from build123d import *

# Parameters (mm, degrees)
SKETCH1_W           = 150
SKETCH1_H           = 120
BOSS_EXTRUDE1_DEPTH = 100
FILLET1_R           = 10
SHELL1_START        = -65
SHELL1_OUTLINE_W    = 90
SHELL1_OUTLINE_H    = 100
SHELL1_DEPTH        = 130
FILLET2_R           = 10
CUT_EXTRUDE1_DEPTH  = 37.5
BOSS_EXTRUDE2_START = 90
BOSS_EXTRUDE2_DEPTH = 90
SKETCH3_W           = 114.3
SKETCH3_H           = 50.8
CUT_EXTRUDE2_DEPTH  = 5.5
FILLET3_R           = 10


# Read off the part's stored shape, not the designer's step: Shell1
with BuildPart() as part:
    # Sketch1 → Boss-Extrude1 (new body)
    with BuildSketch(Plane(origin=(0, 0, 0), x_dir=(1, 0, 0), z_dir=(0, 1, 0))):
        Rectangle(SKETCH1_W, SKETCH1_H)
    extrude(amount=BOSS_EXTRUDE1_DEPTH)

    # Fillet1
    fillet1_edges = [part.edges().sort_by_distance(p)[0] for p in [
        (0, 0, 60),
        (-75, 0, 0),
        (0, 0, -60),
        (75, 0, 0),
        (75, 50, 60),
        (-75, 50, 60),
        (-75, 50, -60),
        (75, 50, -60),
    ]]
    fillet(fillet1_edges, radius=FILLET1_R)

    # Shell1 outline → Shell1 (cut)
    with BuildSketch(Plane.YZ.offset(SHELL1_START)):
        with Locations((55, 0)):
            Rectangle(SHELL1_OUTLINE_W, SHELL1_OUTLINE_H)
    extrude(amount=SHELL1_DEPTH, mode=Mode.SUBTRACT)

    # Fillet2
    fillet2_edges = [part.edges().sort_by_distance(p)[0] for p in [
        (65, 55, -50),
        (-65, 55, -50),
        (-65, 55, 50),
        (65, 55, 50),
    ]]
    fillet(fillet2_edges, radius=FILLET2_R)

    # Sketch2 → Cut-Extrude1 (cut, symmetric)
    with BuildSketch(Plane(origin=(0, 50, 0), x_dir=(1, 0, 0), z_dir=(0, 1, 0))):
        with BuildLine():
            Line((-75, 50), (-75, 0))
            Line((-75, 0), (-70, 0))
            Line((-70, 0), (-70, 40))
            ThreePointArc((-70, 40), (-65.606601718, 50.606601718), (-55, 55))
            Line((-55, 55), (55, 55))
            ThreePointArc((55, 55), (65.606601718, 50.606601718), (70, 40))
            Line((70, 40), (70, 0))
            Line((70, 0), (75, 0))
            Line((75, 0), (75, 50))
            ThreePointArc((75, 50), (72.071067812, 57.071067812), (65, 60))
            Line((65, 60), (-65, 60))
            ThreePointArc((-65, 60), (-72.071067812, 57.071067812), (-75, 50))
        make_face()
    extrude(amount=CUT_EXTRUDE1_DEPTH, both=True, mode=Mode.SUBTRACT)

    # Sketch4 → Boss-Extrude2 (add)
    with BuildSketch(Plane(origin=(0, 10, 0), x_dir=(1, 0, 0), z_dir=(0, 1, 0)).offset(BOSS_EXTRUDE2_START)):
        with BuildLine():
            Line((-65, 40), (65, 40))
            ThreePointArc((65, 40), (62.071067812, 47.071067812), (55, 50))
            Line((55, 50), (-55, 50))
            ThreePointArc((-55, 50), (-62.071067812, 47.071067812), (-65, 40))
        make_face()
    extrude(amount=-BOSS_EXTRUDE2_DEPTH)

    # Sketch3 → Cut-Extrude2 (cut, symmetric)
    with BuildSketch(Plane(origin=(0, 0, -55), x_dir=(-1, 0, 0), z_dir=(0, 0, -1))):
        with Locations((0, 62.1)):
            Rectangle(SKETCH3_W, SKETCH3_H)
    extrude(amount=CUT_EXTRUDE2_DEPTH, both=True, mode=Mode.SUBTRACT)

    # Fillet3
    fillet3_edges = [part.edges().sort_by_distance(p)[0] for p in [
        (-65, 55, -40),
        (65, 55, -40),
    ]]
    fillet(fillet3_edges, radius=FILLET3_R)


solid = part.part
Read the model definition and answer for the solid it produces. Units are mm, in the model's axes. A direction names the side the tool comes from. Round coordinates to 2 decimals unless told otherwise and drop trailing zeros. Order: outer loops, then holes, each group sorted by start corner. A loop starts at its lowest first (then second) coordinate and runs counter-clockwise, first axis right, second up. Notation, with made-up numbers: (89.25, 25) - (138.25, 25) arc R15 ccw to (138.25, 40) - close; hole circle Ø8 at (33, 82.5). An arc over 180 degrees is marked (long way). Use one line per item in the form item = value. Start each with the question number.
(1) For faces 1 (the face through (-57.15, 62, -52)), 2 (the face through (70, 51, -20)), 3 (the face through (-1, 10, 4)), 4 (the face through (-1, 25, -55)), 5 (the face through (-73, 51, 0)), determine the directions among +Z, -Z, +X, -X, +Y, -Y from which every point of the face is accessible in a straight line to the end or side of a thin tool.
(2) The part is cut by section D-D (x = 62.5). Give the vertices of the cut face in (y, z).
(3) The part is cut by section C-C (z = 24.5). Give the vertices of the cut face in (x, y), then the cut area to 3 significant figures.
(4) Find the intervals of material crossed by line 1 along Z through (x, y) = (-15, 25); line 2 along X through (y, z) = (41.5, 7); line 3 along Z through (x, y) = (53, 84), in increasing order. Write a range as from..to.
(5) Flat-ended cylindrical pins translate along their axes: pin 1 Ø6 at (y, z) = (56, -51.5) entering from -X; pin 2 Ø1 at (x, y) = (-50, 48.5) entering from -Z; pin 3 Ø5 at (x, z) = (-42.5, -16) entering from +Y. Find the tip coordinate at first contact, or state that the pin passes through.
(6) Determine the mould class of faces 6 (the face through (-1, 56, -40)), 7 (the face through (72.15, 3.01, -0.7)), 8 (the face through (65.49, 50.52, -50.72)) for opening direction Z: +Z half, -Z half, draft (parallel to the pull), parting line (faces both ways), or undercut.
(7) The part is cut by section A-A (y = 55). Give the vertices of the cut face in (x, z), then the cut area to 3 significant figures.
(8) The part is cut by section B-B (x = 45). Give the vertices of the cut face in (y, z).
Checked values:
q1.face_1 = -Z
q1.face_2 = -Z, +X
q1.face_3 = +Y
q1.face_4 = -Z, +X, -X
q1.face_5 = -Z, -X
q2.outline = (0, -50) arc R10 ccw to (10, -60) - (12.5, -60) - (12.5, -52.99) - (87.5, -52.99) - (87.5, -60) - (100, -60) - (100, -36.61) - (10, -36.61) - (10, 46.61) - (100, 46.61) - (100, 60) - (10, 60) arc R10 ccw to (0, 50) - close
q3.outline = (-75, 10) arc R10 ccw to (-65, 0) - (65, 0) arc R10 ccw to (75, 10) - (75, 100) - (65, 100) - (65, 10) - (-65, 10) - (-65, 100) - (-75, 100) - close
q3.area = 3,260 mm^2
q4.line_1 = -55..-40, 50..60
q4.line_2 = -75..-65, 65..75
q4.line_3 = -49.5..-40, 50..60
q5.pin_1 = -67.36
q5.pin_2 = -49.5
q5.pin_3 = 10
q6.face_6 = undercut
q6.face_7 = draft
q6.face_8 = -Z half
q7.outline = (-75, 0) - (-70, 0) - (-70, -40) arc R15 ccw to (-57.15, -54.85) - (-57.15, -49.5) - (57.15, -49.5) - (57.15, -54.85) arc R15 ccw to (70, -40) - (70, 0) - (75, 0) - (75, 50) arc R10 ccw to (65, 60) - (-65, 60) arc R10 ccw to (-75, 50) - close; hole (-65, -30) arc R10 ccw to (-55, -40) - (55, -40) arc R10 ccw to (65, -30) - (65, 40) arc R10 ccw to (55, 50) - (-55, 50) arc R10 ccw to (-65, 40) - close
q7.area = 4,320 mm^2
q8.outline = (0, -50) arc R10 ccw to (10, -60) - (12.5, -60) - (12.5, -55) - (36.7, -55) - (36.7, -49.5) - (87.5, -49.5) - (87.5, -60) - (100, -60) - (100, -40) - (10, -40) - (10, 50) - (100, 50) - (100, 60) - (10, 60) arc R10 ccw to (0, 50) - close
